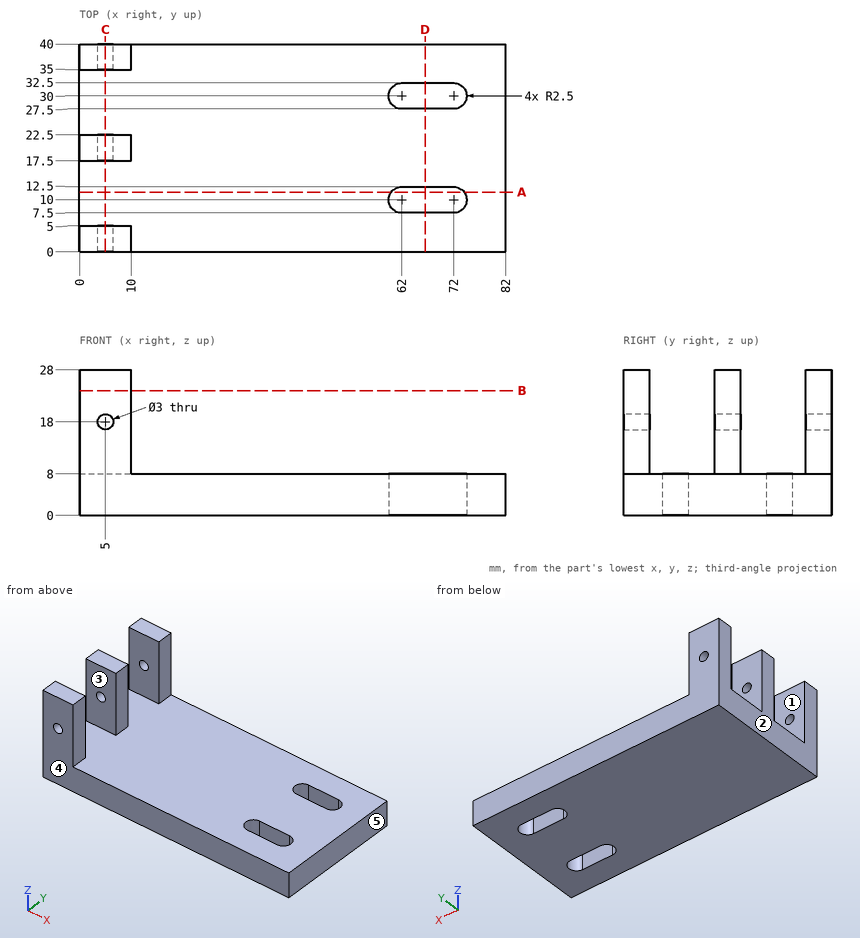
The drawing under review shows one solid part. Ordinate dimensions are in mm from its lowest x, y, z. A direction names the side the tool comes from. Round coordinates to 2 decimals unless told otherwise and drop trailing zeros. Order: outer loops, then holes, each group sorted by start corner. A loop starts at its lowest first (then second) coordinate and runs counter-clockwise, first axis right, second up. Notation, with made-up numbers: M -9,73.5 L 27,73.5 A17 ccw 27,101.5 Z; hole C 74,17 d10. An arc over 180 degrees is marked long. Answer as CSV lines item,"result". Start each with the question number.
1) Wall thickness on line 1 along Y through (x, z) = (7, 17.75); line 2 along X through (y, z) = (38.85, 18); line 3 along Z through (x, y) = (9, 23.5): over which ranges is each line inside the solid? List them lowest first. Write a range as [from, to].
2) Add section B-B (z = 24). Give the boundary of the cut face in (x, y), then the cut area to 3 significant figures.
3) Tool access review of the marked faces 1 and 2: name each direction out of +Z, -Z, +X, -X, +Y, -Y from which nothing blocks a thin tool from reaching the whole face with its end or side.
4) Add section A-A (y = 11.5). Give the boundary of the cut face in (x, z).
5) Add section C-C (x = 5). Give the boundary of the cut face in (y, z).
6) The part is to be moulded in two halves that separate along Y. For the marked faces 3, 4 and 5, say which applies: +Y half, -Y half, draft (parallel to the pull), parting line (faces both ways), or undercut.
7) For pin 1 Ø2.5 at (x, z) = (5, 18) entering from +Y; pin 2 Ø20 at (x, y) = (26.5, 17) entering from +Z; pin 3 Ø5.5 at (y, z) = (2, 18.5) entering from +X, all flat-tipped, find the tip position at first contact; note any pin that passes through.
8) Add section D-D (x = 66.5). Give the boundary of the cut face in (y, z).
Resolved:
1,line 1,"[0, 5], [17.5, 22.5], [35, 40]"
1,line 2,"[0, 3.5], [6.5, 10]"
1,line 3,"[0, 8]"
2,outline,"M 0,0 L 10,0 L 10,5 L 0,5 Z; M 0,17.5 L 10,17.5 L 10,22.5 L 0,22.5 Z; M 0,35 L 10,35 L 10,40 L 0,40 Z"
2,area,"150 mm^2"
3,face 1,"+Z, +X, -X"
3,face 2,"+Z, -Z, -X, +Y, -Y"
4,outline,"M 0,0 L 60,0 L 60,8 L 0,8 Z; M 74,0 L 82,0 L 82,8 L 74,8 Z"
5,outline,"M 0,0 L 40,0 L 40,16.5 L 35,16.5 L 35,8 L 22.5,8 L 22.5,16.5 L 17.5,16.5 L 17.5,8 L 5,8 L 5,16.5 L 0,16.5 Z; M 0,19.5 L 5,19.5 L 5,28 L 0,28 Z; M 17.5,19.5 L 22.5,19.5 L 22.5,28 L 17.5,28 Z; M 35,19.5 L 40,19.5 L 40,28 L 35,28 Z"
6,face 3,"undercut"
6,face 4,"-Y half"
6,face 5,"draft"
7,pin 1,"through"
7,pin 2,"z = 8"
7,pin 3,"x = 10"
8,outline,"M 0,0 L 7.5,0 L 7.5,8 L 0,8 Z; M 12.5,0 L 27.5,0 L 27.5,8 L 12.5,8 Z; M 32.5,0 L 40,0 L 40,8 L 32.5,8 Z"
